from build123d import *

# Parameters (mm, degrees)
BASIC_SHAPE_SKETCH_R                = 46.96825
BASIC_SHAPE_SKETCH_R_2              = 24.53175
BASIC_SHAPE_DEPTH                   = 4.8
BATTERY_SLOT_SKETCH_R               = 9.65
BATTERY_SLOT_DEPTH                  = 3.3
BATTERY_SLOT_PATTERN_COUNT          = 5
BATTERY_SLOT_PATTERN_ANGLE          = 130.88
BATTERY_SLOT_MIRROR_COPY_1_SKETCH_R = 9.65
BATTERY_SLOT_MIRROR_COPY_1_DEPTH    = 3.3
BATTERY_SLOT_MIRROR_COPY_2_SKETCH_R = 9.65
BATTERY_SLOT_MIRROR_COPY_2_DEPTH    = 3.3
BATTERY_SLOT_MIRROR_COPY_3_SKETCH_R = 9.65
BATTERY_SLOT_MIRROR_COPY_3_DEPTH    = 3.3
BATTERY_SLOT_MIRROR_COPY_4_SKETCH_R = 9.65
BATTERY_SLOT_MIRROR_COPY_4_DEPTH    = 3.3
SLIT_DEPTH                          = 67.596343865
BUS_SLIT_DEPTH                      = 3.3
CAP_2_DEPTH                         = 2
PLUNGER_DEPTH                       = 66.5
PLUNGER_CAVITY_DEPTH                = 66.5
LIP_DEPTH                           = 2
EXTRA_CUT_DEPTH                     = 94.990866663
BARRIERS_DEPTH                      = 51.5
SKETCH15_W                          = 10
SKETCH15_H                          = 8
CUT_EXTRUDE6_DEPTH                  = 96.416366605


with BuildPart() as part:
    # Basic_Shape_Sketch → Basic_Shape (new body)
    with BuildSketch(Plane.XY):
        Circle(BASIC_SHAPE_SKETCH_R)
        Circle(BASIC_SHAPE_SKETCH_R_2, mode=Mode.SUBTRACT)
    extrude(amount=BASIC_SHAPE_DEPTH)

    # Battery_Slot_Sketch → Battery_Slot (cut)
    with BuildSketch(Plane.XY.offset(4.8)):
        with Locations((-10.069761866, -34.302512969)):
            Circle(BATTERY_SLOT_SKETCH_R)
    battery_slot = extrude(amount=-BATTERY_SLOT_DEPTH, mode=Mode.SUBTRACT)

    # Battery_Slot_Pattern: Battery_Slot ×5 about axis
    battery_slot_pattern_axis = Axis((0, 0, 0), (0, 0, -1))
    for i in range(1, BATTERY_SLOT_PATTERN_COUNT):
        add(battery_slot.rotate(battery_slot_pattern_axis, i * BATTERY_SLOT_PATTERN_ANGLE / (BATTERY_SLOT_PATTERN_COUNT - 1)), mode=Mode.SUBTRACT)

    # Battery_Slot_Mirror: Battery_Slot across plane
    add(battery_slot.mirror(Plane(origin=(0, 0, 0), x_dir=(0, 0, 1), z_dir=(1, 0, 0))), mode=Mode.SUBTRACT)

    # Battery_Slot_Mirror copy 1 sketch → Battery_Slot_Mirror copy 1 (cut)
    with BuildSketch(Plane(origin=(0, 0, 4.8), x_dir=(-0.8413221512344797, -0.5405340302350882, 0), z_dir=(0, 0, 1))):
        with Locations((-10.069761866, 34.302512969)):
            Circle(BATTERY_SLOT_MIRROR_COPY_1_SKETCH_R)
    extrude(amount=-BATTERY_SLOT_MIRROR_COPY_1_DEPTH, mode=Mode.SUBTRACT)

    # Battery_Slot_Mirror copy 2 sketch → Battery_Slot_Mirror copy 2 (cut)
    with BuildSketch(Plane(origin=(0, 0, 4.8), x_dir=(-0.4156459243156256, -0.9095265062656553, 0), z_dir=(0, 0, 1))):
        with Locations((-10.069761866, 34.302512969)):
            Circle(BATTERY_SLOT_MIRROR_COPY_2_SKETCH_R)
    extrude(amount=-BATTERY_SLOT_MIRROR_COPY_2_DEPTH, mode=Mode.SUBTRACT)

    # Battery_Slot_Mirror copy 3 sketch → Battery_Slot_Mirror copy 3 (cut)
    with BuildSketch(Plane(origin=(0, 0, 4.8), x_dir=(0.14193790484034807, -0.9898755634773152, 0), z_dir=(0, 0, 1))):
        with Locations((-10.069761866, 34.302512969)):
            Circle(BATTERY_SLOT_MIRROR_COPY_3_SKETCH_R)
    extrude(amount=-BATTERY_SLOT_MIRROR_COPY_3_DEPTH, mode=Mode.SUBTRACT)

    # Battery_Slot_Mirror copy 4 sketch → Battery_Slot_Mirror copy 4 (cut)
    with BuildSketch(Plane(origin=(0, 0, 4.8), x_dir=(0.6544769311996185, -0.7560819707726999, 0), z_dir=(0, 0, 1))):
        with Locations((-10.069761866, 34.302512969)):
            Circle(BATTERY_SLOT_MIRROR_COPY_4_SKETCH_R)
    extrude(amount=-BATTERY_SLOT_MIRROR_COPY_4_DEPTH, mode=Mode.SUBTRACT)

    # Slit_Sketch → Slit (cut, through all)
    with BuildSketch(Plane.XY.offset(4.8)):
        with BuildLine():
            Line((-8.33, 46.223669349), (-8.33, 23.074181634))
            Line((-8.33, 23.074181634), (8.33, 23.074181634))
            Line((8.33, 23.074181634), (8.33, 46.223669349))
            ThreePointArc((8.33, 46.223669349), (0, 54.553669349), (-8.33, 46.223669349))
        make_face()
    extrude(amount=-SLIT_DEPTH, mode=Mode.SUBTRACT)

    # Bus_Slit_Sketch → Bus_Slit (cut)
    with BuildSketch(Plane.XY.offset(4.8)):
        with BuildLine():
            ThreePointArc((-9.754463235, 31.132636766), (0, -32.625), (9.754463235, 31.132636766))
            ThreePointArc((9.754463235, 31.132636766), (10.629095474, 34.20551129), (12.459123069, 36.824392423))
            ThreePointArc((12.459123069, 36.824392423), (0, -38.875), (-12.459123069, 36.824392423))
            ThreePointArc((-12.459123069, 36.824392423), (-10.629095474, 34.20551129), (-9.754463235, 31.132636766))
        make_face()
    extrude(amount=-BUS_SLIT_DEPTH, mode=Mode.SUBTRACT)

    # Cap_2_Sketch → Cap_2 (add)
    with BuildSketch(Plane(origin=(0, 0, 0), x_dir=(-1, 0, 0), z_dir=(0, 0, -1))):
        with BuildLine():
            Line((-8.33, 34.648925491), (-8.33, 23.074181634))
            Line((-8.33, 23.074181634), (8.33, 23.074181634))
            Line((8.33, 23.074181634), (8.33, 34.648925491))
            ThreePointArc((8.33, 34.648925491), (0, -35.636174566), (-8.33, 34.648925491))
        make_face()
    extrude(amount=CAP_2_DEPTH)

    # Sketch1 → Plunger (add)
    with BuildSketch(Plane.XY):
        with BuildLine():
            Line((-7.5, 8.074181634), (7.5, 8.074181634))
            Line((7.5, 8.074181634), (8.154017112, 19.893767993))
            ThreePointArc((8.154017112, 19.893767993), (0, -21.5), (-8.154017112, 19.893767993))
            Line((-8.154017112, 19.893767993), (-7.5, 8.074181634))
        make_face()
    extrude(amount=PLUNGER_DEPTH)

    # Sketch11 → Plunger Cavity (cut)
    with BuildSketch(Plane(origin=(0, 0, -2), x_dir=(-1, 0, 0), z_dir=(0, 0, -1))):
        with BuildLine():
            Line((-8.61374371, 19.152112659), (-7.973098193, 7.574181634))
            Line((-7.973098193, 7.574181634), (7.973098193, 7.574181634))
            Line((7.973098193, 7.574181634), (8.61374371, 19.152112659))
            ThreePointArc((8.61374371, 19.152112659), (0, -21), (-8.61374371, 19.152112659))
        make_face()
    extrude(amount=-PLUNGER_CAVITY_DEPTH, mode=Mode.SUBTRACT)

    # Sketch10 → Lip (add)
    with BuildSketch(Plane(origin=(0, 0, -2), x_dir=(-1, 0, 0), z_dir=(0, 0, -1))):
        with BuildLine():
            Line((-8.33, 34.648925491), (-8.33, 32.648925491))
            ThreePointArc((-8.33, 32.648925491), (0, -33.694825059), (8.33, 32.648925491))
            Line((8.33, 32.648925491), (8.33, 34.648925491))
            ThreePointArc((8.33, 34.648925491), (0, -35.636174566), (-8.33, 34.648925491))
        make_face()
    extrude(amount=LIP_DEPTH)

    # Sketch12 → Extra_Cut (cut, through all)
    with BuildSketch(Plane.XY):
        Polygon((-7.5, 8.074181634), (-8.33, 23.074181634), (8.33, 23.074181634), (7.5, 8.074181634), align=None)
    extrude(amount=-EXTRA_CUT_DEPTH, mode=Mode.SUBTRACT)

    # Sketch14 → Barriers (add)
    with BuildSketch(Plane(origin=(0, 0, 13), x_dir=(-1, 0, 0), z_dir=(0, 0, -1))):
        with BuildLine():
            Line((-8.094524385, 9.768630899), (-12.482303066, -16.88763187))
            ThreePointArc((-12.482303066, -16.88763187), (-12.256826493, -17.051985349), (-12.029186165, -17.213328562))
            Line((-12.029186165, -17.213328562), (-10.771652468, -9.573665961))
            Line((-10.771652468, -9.573665961), (10.771652468, -9.573665961))
            Line((10.771652468, -9.573665961), (12.029186165, -17.213328562))
            ThreePointArc((12.029186165, -17.213328562), (12.256826493, -17.051985349), (12.482303066, -16.88763187))
            Line((12.482303066, -16.88763187), (8.094524385, 9.768630899))
            Line((8.094524385, 9.768630899), (7.959093124, 7.574181634))
            Line((7.959093124, 7.574181634), (10.699314208, -9.072978255))
            Line((10.699314208, -9.072978255), (-10.699314208, -9.072978255))
            Line((-10.699314208, -9.072978255), (-7.959093124, 7.574181634))
            Line((-7.959093124, 7.574181634), (-8.094524385, 9.768630899))
        make_face()
    extrude(amount=-BARRIERS_DEPTH)

    # Sketch15 → Cut-Extrude6 (cut, through all)
    with BuildSketch(Plane(origin=(0, 0, 64.5), x_dir=(-1, 0, 0), z_dir=(0, 0, -1))):
        Polygon((-16.676224256, 7.812290296), (-8.782450836, 6.512928453), (-10.40665314, -3.354288322), (-18.30042656, -2.054926479), align=None)
        Polygon((8.782450836, 6.512928453), (16.676224256, 7.812290296), (18.30042656, -2.054926479), (10.40665314, -3.354288322), align=None)
        with Locations((0, -4.922978255)):
            Rectangle(SKETCH15_W, SKETCH15_H)
        with Locations((0, -13.723665961)):
            Rectangle(SKETCH15_W, SKETCH15_H)
    extrude(amount=-CUT_EXTRUDE6_DEPTH, mode=Mode.SUBTRACT)


solid = part.part
CAD build for the part. Positions are in the model's coordinates, mm. A direction names the side the tool comes from. Give positions to 0.01 mm unless a question says otherwise; leave off trailing zeros. Loops run counter-clockwise (first coordinate to the right, second up) from the corner with the lowest first, then second, coordinate; pieces in that order, holes last. Notation, with made-up numbers: M 1,-2.5 L 39,-2.5 A19 ccw 39,11.5 Z; hole C 53.25,85.25 d1. An arc over 180 degrees is marked long. Answer in a Markdown table with one row per item. Add a question column.
Item 1: Band-saw the part on C-C on y = 1. Give the number of separate pieces and of enclosed holes in the cut face, then the cut area to 3 significant figures.
Item 2: Band-saw the part on B-B on z = 10. Give the cut face in (x, y), then the cut area to 3 significant figures.
Item 3: Band-saw the part on A-A on z = 33. Give the cut face in (x, y).
Item 4: Drop flat-ended pins along their axis: P1, Ø1, axis at y = -1.5, z = 7.5, coming from the -X side; P2, Ø4, axis at y = -28.5, z = 5, coming from the -X side; P3, Ø20, axis at x = 5, y = -2, coming from the -Z side. Give the stop position or say it passes through.
Item 5: Mould opens along Y. For faces 3 (the face through (-1.948, -46.928, 2.366)), 4 (the face through (-23.81, 10.696, 3.173)), 5 (the face through (0, 8.074, 33)) say: +Y half, -Y half, draft (parallel to the pull), parting line (faces both ways), or undercut.
Item 6: Probe probe 1 along X at (y, z) = (0, 1.05); probe 2 along X at (y, z) = (0, -3); probe 3 along Y at (x, z) = (13, 3.5). List the from-to ranges inside material, lowest first.
Item 7: Tool access for faces 1 (the face through (38.48, 5.54, 3.17)), 2 (the face through (-10.32, -3.75, 38.39)): list every direction of +Z, -Z, +X, -X, +Y, -Y with a clear straight run to the whole face (end or side of a thin tool).
Reply:
| question | item | result |
|---|---|---|
| 1 | separate pieces | 3 |
| 1 | enclosed holes | 0 |
| 1 | area | 352 mm^2 |
| 2 | outline | M -8.15,19.89 A21.5 ccw long 8.15,19.89 L 7.5,8.07 L -7.5,8.07 Z; hole M -8.61,19.15 A21 ccw long 8.61,19.15 L 7.97,7.57 L -7.97,7.57 Z |
| 2 | area | 77.6 mm^2 |
| 3 | outline | M -8.15,19.89 A21.5 ccw long 8.15,19.89 L 7.5,8.07 L -7.5,8.07 Z; hole M -12.48,-16.89 L -8.09,9.77 L -8.61,19.15 A21 ccw Z; hole M -12.03,-17.21 A21 ccw 12.03,-17.21 L 10.77,-9.57 L -10.77,-9.57 Z; hole M -10.7,-9.07 L 10.7,-9.07 L 7.96,7.57 L -7.96,7.57 Z; hole M 8.09,9.77 L 12.48,-16.89 A21 ccw 8.61,19.15 Z |
| 4 | P1 | stops at x = -21.48 |
| 4 | P2 | stops at x = -38.77 |
| 4 | P3 | stops at z = -2 |
| 5 | face 3 | parting line |
| 5 | face 4 | undercut |
| 5 | face 5 | +Y half |
| 6 | probe 1 | x = -46.97 to -24.53, -21.5 to -21, 21 to 21.5, 24.53 to 46.97 |
| 6 | probe 2 | x = -35.64 to -33.69, 33.69 to 35.64 |
| 6 | probe 3 | y = -45.13 to -43.5, -25.11 to -20.8, -17.12 to -16.49, 16.49 to 17.12, 20.8 to 22.79, 37.33 to 45.13 |
| 7 | face 1 | +Z |
| 7 | face 2 | -Z |
